```python
from build123d import *

# Parameters (mm, degrees)
BOSS_EXTRUDE4_DEPTH = 1.27
SKETCH11_R          = 11.402996403
BOSS_EXTRUDE6_DEPTH = 33.02
SKETCH12_W          = 22.792557874
SKETCH12_H          = 15.82816519
CUT_EXTRUDE4_DEPTH  = 12.7
FILLET1_R           = 2.54
SKETCH13_W          = 31.831001044
SKETCH13_H          = 0.811195954
SKETCH13_W_2        = 43.310342169
SKETCH13_H_2        = 1.569408792
CUT_EXTRUDE5_DEPTH  = 22.86


with BuildPart() as part:
    # Sketch2 → Boss-Extrude4 (new body)
    with BuildSketch(Plane(origin=(0, 0, 0), x_dir=(1, 0, 0), z_dir=(0, 1, 0))):
        with BuildLine():
            Line((-42.31395881, 38.1), (59.28604119, 38.1))
            ThreePointArc((59.28604119, 38.1), (97.38604119, 0), (59.28604119, -38.1))
            Line((59.28604119, -38.1), (-42.31395881, -38.1))
            ThreePointArc((-42.31395881, -38.1), (-80.41395881, 0), (-42.31395881, 38.1))
        make_face()
    extrude(amount=BOSS_EXTRUDE4_DEPTH)

    # Sketch11 → Boss-Extrude6 (add)
    with BuildSketch(Plane(origin=(0, 1.27, 0), x_dir=(1, 0, 0), z_dir=(0, 1, 0))):
        with Locations(Location((59.460873827, 0, 0), (0, 0, 270))):
            Circle(SKETCH11_R)
    extrude(amount=BOSS_EXTRUDE6_DEPTH)

    # Sketch12 → Cut-Extrude4 (cut)
    with BuildSketch(Plane(origin=(0, 1.27, 0), x_dir=(1, 0, 0), z_dir=(0, 1, 0))):
        with Locations((-34.122794633, -1.569408792)):
            Rectangle(SKETCH12_W, SKETCH12_H)
    extrude(amount=-CUT_EXTRUDE4_DEPTH, mode=Mode.SUBTRACT)

    # Fillet1
    # the kernel refuses this fillet: 2.54 mm, written as the material it takes off along each edge
    with BuildSketch(Plane(origin=(-42.31395881, 0, 0), x_dir=(0, 0, 1), z_dir=(1, 0, 0))) as fillet1_piece_1:
        with BuildLine():
            CenterArc((35.900295474, -2.54), FILLET1_R, 30, 60)
            Line((35.900295474, 0), (35.900295474, 0.0508))
            Line((35.900295474, 0.0508), (38.1, 0.0508))
            Line((38.1, 0.0508), (38.1508, 0))
            ThreePointArc((38.1508, 0), (38.1508, -0.635), (38.143994091, -1.2446))
            Line((38.143994091, -1.2446), (38.1, -1.27))
        make_face()
    revolve(axis=Axis((-42.31395881, 0, 0), (0, -1, 0)), revolution_arc=180, mode=Mode.SUBTRACT)
    with BuildSketch(Plane(origin=(59.28604119, 0, 38.1), x_dir=(0, 1, 0), z_dir=(-1, 0, 0))) as fillet1_piece_2:
        with BuildLine():
            CenterArc((2.54, 2.199704526), FILLET1_R, 180, 60)
            Line((0, 2.199704526), (-0.0508, 2.199704526))
            Line((-0.0508, 2.199704526), (-0.0508, 0))
            Line((-0.0508, 0), (0, -0.0508))
            ThreePointArc((0, -0.0508), (0.635, -0.0508), (1.2446, -0.043994091))
            Line((1.2446, -0.043994091), (1.27, 0))
        make_face()
    extrude(amount=101.6, mode=Mode.SUBTRACT)
    with BuildSketch(Plane(origin=(59.28604119, 0, 0), x_dir=(0, 0, -1), z_dir=(-1, 0, 0))) as fillet1_piece_3:
        with BuildLine():
            CenterArc((35.900295474, -2.54), FILLET1_R, 30, 60)
            Line((35.900295474, 0), (35.900295474, 0.0508))
            Line((35.900295474, 0.0508), (38.1, 0.0508))
            Line((38.1, 0.0508), (38.1508, 0))
            ThreePointArc((38.1508, 0), (38.1508, -0.635), (38.143994091, -1.2446))
            Line((38.143994091, -1.2446), (38.1, -1.27))
        make_face()
    revolve(axis=Axis((59.28604119, 0, 0), (0, -1, 0)), revolution_arc=180, mode=Mode.SUBTRACT)
    with BuildSketch(Plane(origin=(-42.31395881, 0, -38.1), x_dir=(0, 0, 1), z_dir=(1, 0, 0))) as fillet1_piece_4:
        with BuildLine():
            CenterArc((2.199704526, -2.54), FILLET1_R, 90, 60)
            Line((0, -1.27), (-0.043994091, -1.2446))
            ThreePointArc((-0.043994091, -1.2446), (-0.0508, -0.635), (-0.0508, 0))
            Line((-0.0508, 0), (0, 0.0508))
            Line((0, 0.0508), (2.199704526, 0.0508))
            Line((2.199704526, 0.0508), (2.199704526, 0))
        make_face()
    extrude(amount=101.6, mode=Mode.SUBTRACT)

    # Sketch13 → Cut-Extrude5 (cut)
    with BuildSketch(Plane.XZ):
        with Locations((-61.546134254, 0.405597977)):
            Rectangle(SKETCH13_W, SKETCH13_H)
        with Locations((0.488633532, 0.784704396)):
            Rectangle(SKETCH13_W_2, SKETCH13_H_2)
    extrude(amount=-CUT_EXTRUDE5_DEPTH, mode=Mode.SUBTRACT)


solid = part.part
```
For this review, take the finished solid that the model builds, in its own axes (mm). A direction names the side the tool comes from. Give positions to 0.01 mm unless a question says otherwise; leave off trailing zeros. Order: outer loops, then holes, each group sorted by start corner. A loop starts at its lowest first (then second) coordinate and runs counter-clockwise, first axis right, second up.
1) Take a section at A-A (x = 4). Give the boundary of the cut face in (y, z), then the cut area to 3 significant figures.
2) Take a section at B-B (x = -26.5). Give the boundary of the cut face in (y, z).
3) Take a section at C-C (y = 13.5). Give the boundary of the cut face in (x, z).
4) Insertion check: pin 1 (1 mm diameter, centred on y = 0.5, z = 1, fed in from -X); pin 2 (1.4 mm diameter, centred on x = -32.5, y = 0.5, fed in from -Z); pin 3 (0.6 mm diameter, centred on y = 1, z = 5, fed in from +X). Each pin has a flat end and moves straight along its axis. Give the tip position at first contact, or say it passes through.
5) Wall thickness on line 1 (Y direction, x = 77, z = 25); line 2 (X direction, y = 18.5, z = 9.5); line 3 (X direction, y = 6.5, z = 8): over which ranges is each line inside the solid? List them lowest first.
6) For faces 1 (the face through (48.33, 17.55, -2.47)), 2 (the face through (10, 0, -1)), list the 3-axis set-ups (+Z, -Z, +X, -X, +Y, -Y) from which the entire face can be reached by the end or side of a thin tool; tool diameter is ignored.
Derived:
1. outline: (0, -35.9) arc R2.54 ccw to (1.27, -38.1) - (1.27, 0) - (0, 0) - close; (0, 1.57) - (1.27, 1.57) - (1.27, 38.1) arc R2.54 ccw to (0, 35.9) - close
1. area: 93.2 mm2
2. outline: (0, -35.9) arc R2.54 ccw to (1.27, -38.1) - (1.27, -6.34) - (0, -6.34) - close; (0, 9.48) - (1.27, 9.48) - (1.27, 38.1) arc R2.54 ccw to (0, 35.9) - close
3. outline: circle Ø22.81 at (59.46, 0)
4. pin 1: stops at x = -80.22
4. pin 2: stops at z = -38.06
4. pin 3: stops at x = 97.07
5. line 1: y = 0 to 1.27
5. line 2: x = 53.15 to 65.77
5. line 3: x = 51.34 to 67.59
6. face 1: +Y
6. face 2: +Z, -Z, +X, -X, -Y
